Check sheet for the modelled part. Datum: model origin and axes. Units: mm. A direction names the side the tool comes from. Round coordinates to 2 decimals unless told otherwise and drop trailing zeros. Order: outer loops, then holes, each group sorted by start corner. A loop starts at its lowest first (then second) coordinate and runs counter-clockwise, first axis right, second up. Notation, with made-up numbers: (84, -21.75) -> (96, -21.75) arc R19 cw to (96, -9.75) -> close; hole circle Ø1 at (47, 86). An arc over 180 degrees is marked (long way). Answer in a Markdown table with one row per item.
from build123d import *

# Parameters (mm, degrees)
SKETCH2_R           = 9
BOSS_EXTRUDE1_DEPTH = 9
SKETCH3_R           = 4
CUT_EXTRUDE1_DEPTH  = 7
SKETCH4_R           = 9
SKETCH4_R_2         = 7
CUT_EXTRUDE2_DEPTH  = 8


with BuildPart() as part:
    # Sketch2 → Boss-Extrude1 (new body)
    with BuildSketch(Plane.XY):
        Circle(SKETCH2_R)
    extrude(amount=BOSS_EXTRUDE1_DEPTH)

    # Sketch3 → Cut-Extrude1 (cut)
    with BuildSketch(Plane.XY.offset(9)):
        Circle(SKETCH3_R)
    extrude(amount=-CUT_EXTRUDE1_DEPTH, mode=Mode.SUBTRACT)

    # Sketch4 → Cut-Extrude2 (cut)
    with BuildSketch(Plane(origin=(0, 0, 0), x_dir=(-1, 0, 0), z_dir=(0, 0, -1))):
        Circle(SKETCH4_R)
        Circle(SKETCH4_R_2, mode=Mode.SUBTRACT)
    extrude(amount=-CUT_EXTRUDE2_DEPTH, mode=Mode.SUBTRACT)


solid = part.part
Item 1: Depth check by flat-ended pin: P1, Ø4, axis at y = -5.5, z = 1.5, coming from the -X side; P2, Ø3, axis at x = 2.5, z = 2, coming from the +Y side; P3, Ø3, axis at x = 3, z = 8, coming from the +Y side; P4, Ø6.5, axis at x = 1.5, y = -2, coming from the +Z side. Enter the tip coordinate at first touch or a pass-through.
Result sheet:
| item | result |
|---|---|
| P1 | stops at x = -6.06 |
| P2 | stops at y = 6.93 |
| P3 | stops at y = 8.87 |
| P4 | stops at z = 9 |
Item 2: Set-up check for faces 4 (the flat face through (0, 0, 0)), 5 (the flat face through (0, 0, 2)), 6 (the flat face through (0, -7.3, 8)): record each of +Z, -Z, +X, -X, +Y, -Y from which the full face is reachable in a straight line by a thin tool's end or side.
Result sheet:
| item | result |
|---|---|
| face 4 | -Z, +X, -X, +Y, -Y |
| face 5 | +Z |
| face 6 | -Z |
Item 3: Mould release check, pull along X, two halves, no side actions. Record for faces 1 (the flat face through (4, -2, 9)), 2 (the cylindrical face through (-6.466, -2.681, 3.944)), 3 (the cylindrical face through (-0.867, -3.905, 5.549)): pulls with the +X half, pulls with the -X half, needs draft (parallel to the pull), parting line crosses it, or undercut.
Result sheet:
| item | result |
|---|---|
| face 1 | needs draft |
| face 2 | parting line crosses it |
| face 3 | undercut |
Item 4: Cross-section at D-D (x = -6). Record the boundary of the cut face in (y, z).
Result sheet:
| item | result |
|---|---|
| outline | (-6.71, 8) -> (-3.61, 8) -> (-3.61, 0) -> (3.61, 0) -> (3.61, 8) -> (6.71, 8) -> (6.71, 9) -> (-6.71, 9) -> close |
Item 5: Scan lines: line 1 (Y direction, x = 0, z = 5.25); line 2 (Z direction, x = -4.5, y = 5.5); line 3 (Z direction, x = 3.5, y = 0.5). Record each from-to range of solid material in increasing order. Write a range as [from, to].
Result sheet:
| item | result |
|---|---|
| line 1 | y = [-7, -4], [4, 7] |
| line 2 | z = [8, 9] |
| line 3 | z = [0, 2] |
Item 6: Cross-section at C-C (z = 2.5). Record the boundary of the cut face in (x, y).
Result sheet:
| item | result |
|---|---|
| outline | circle Ø14 at (0, 0); hole circle Ø8 at (0, 0) |
Item 7: Cross-section at A-A (x = 0). Record the boundary of the cut face in (y, z), and give its area (3 significant figures).
Result sheet:
| item | result |
|---|---|
| outline | (-9, 8) -> (-7, 8) -> (-7, 0) -> (7, 0) -> (7, 8) -> (9, 8) -> (9, 9) -> (4, 9) -> (4, 2) -> (-4, 2) -> (-4, 9) -> (-9, 9) -> close |
| area | 74.0 mm^2 |
